Geometry: final body of the model. Coordinates: model frame, mm. A direction names the side the tool comes from. Give positions to 0.01 mm unless a question says otherwise; leave off trailing zeros. Write each loop counter-clockwise with the first axis right and the second up, starting at its lowest first coordinate (ties: lowest second). Pieces come first, ordered by that corner, then holes. Notation, with made-up numbers: M 70.5,9.25 L 100.5,9.25 A9 ccw 100.5,22.25 Z; hole C -31.5,-14.75 d11. An arc over 180 degrees is marked long. Use one line per item in the form item = value. Start each with the question number.
Item 1: Section query A-A on z = 3.6. Return loops of the section in (x, y).
Item 2: Access query for faces 4 (the cylindrical face through (5.96, -9.43, 2.4)), 5 (the flat face through (6, -3, 3)), 6 (the cylindrical face through (6.04, 3.43, 2.4)), 7 (the flat face through (0, -3, 3)). Directions: +Z, -Z, +X, -X, +Y, -Y. A direction counts if a zero-diameter tool reaches every point of the face in a straight line with its end or side. Return the directions, or none.
Item 3: Section query B-B on x = 5.5. Return loops of the section in (y, z), then the cut area to 3 significant figures.
Item 4: Section query D-D on z = 2.7. Return loops of the section in (x, y), then the cut area to 3 significant figures.
Item 5: Section query C-C on y = -7.75. Return loops of the section in (x, z), then the cut area to 3 significant figures.
Item 6: Material intervals for line 1 along X through (y, z) = (-3, 4.4); line 2 along Z through (x, y) = (4, 2), sorted ascending. Write a range as from..to.
Item 7: Pull-direction query (X, two-part tool) for faces 1 (the flat face through (8.8, -3, 5)), 2 (the flat face through (12, -3, 3)), 3 (the flat face through (5.9, 4, 0.3)); classes: released by +X, released by -X, zero draft, split by the parting line, or undercut.
Autodesk Inventor part; units mm, degrees
ref_plane "YZ Plane" through (0, 0, 0) normal (1, 0, 0) x (0, 1, 0)
ref_plane "XZ Plane" through (0, 0, 0) normal (0, 1, 0) x (-1, 0, 0)
ref_plane "XY Plane" through (0, 0, 0) normal (0, 0, 1) x (1, 0, 0)
ref_plane "Work Plane1" through (0, 0, 0) normal (0, 0, 1) x (1, 0, 0)
sketch "Sketch1" plane through (0, 0, 0) normal (0, 0, 1) x (1, 0, 0)
  line L0 (12, 0) -> (12, 4)
  line L1 (0, 4) -> (12, 4)
  line L2 (0, 0) -> (0, 4)
  line L3 (12, 0) -> (12, -10)
  line L4 (12, -10) -> (0, -10)
  line L5 (0, -10) -> (0, 4)
  line L6 (0, 4) -> (12, 4)
  line L7 (12, 4) -> (12, 0)
  dimension "d0" = 10
extrude "Extrusion1" add sketch "Sketch1" along normal blind 3
sketch "Sketch2" plane through (0, 0, 3) normal (0, 0, 1) x (1, 0, 0)
  line L0 (12, -10) -> (12, 4)
  line L1 (12, 4) -> (0, 4)
  line L2 (0, 4) -> (0, -10)
  line L3 (0, -10) -> (12, -10)
  line L4 (6, 4) -> (8.8, 4)
  line L5 (6, 4) -> (3.2, 4)
  line L6 (8.8, 4) -> (8.8, -10)
  line L7 (8.8, -10) -> (12, -10)
  line L8 (12, 4) -> (8.8, 4)
  line L9 (3.2, 4) -> (3.2, -10)
  line L10 (3.2, -10) -> (0, -10)
  line L11 (0, -10) -> (0, 4)
  line L12 (0, 4) -> (3.2, 4)
  point P0 (0, 0)
  dimension "d3" = 2.8
  dimension "d4" = 2.8
extrude "Extrusion2" add sketch "Sketch2" along normal blind 3 contours L3 L6 L1 L0 | L3 L2 L1 L9
fillet "Fillet1" radius 2 1 edges at (6, 4, 3)
fillet "Fillet2" radius 2 1 edges at (6, -10, 3)
equation "\"d4\" = d3"
properties part number "commutator_attachement_side_plate"
Answer sheet:
q1.outline = M 0,-10 L 3.2,-10 L 3.2,4 L 0,4 Z; M 8.8,-10 L 12,-10 L 12,4 L 8.8,4 Z
q2.face_4 = +Z, -Y
q2.face_5 = +Z, +Y, -Y
q2.face_6 = +Z, +Y
q2.face_7 = +Z, -Z, -X, +Y, -Y
q3.outline = M -10,0 L 4,0 L 4,1 A2 ccw 2,3 L -8,3 A2 ccw -10,1 Z
q3.area = 40.3 mm2
q4.outline = M 0,-10 L 3.2,-10 L 3.2,-9.05 L 8.8,-9.05 L 8.8,-10 L 12,-10 L 12,4 L 8.8,4 L 8.8,3.05 L 3.2,3.05 L 3.2,4 L 0,4 Z
q4.area = 157 mm2
q5.outline = M 0,0 L 12,0 L 12,6 L 8.8,6 L 8.8,3 L 3.2,3 L 3.2,6 L 0,6 Z
q5.area = 55.2 mm2
q6.line_1 = 0..3.2, 8.8..12
q6.line_2 = 0..3
q7.face_1 = undercut
q7.face_2 = released by +X
q7.face_3 = zero draft
